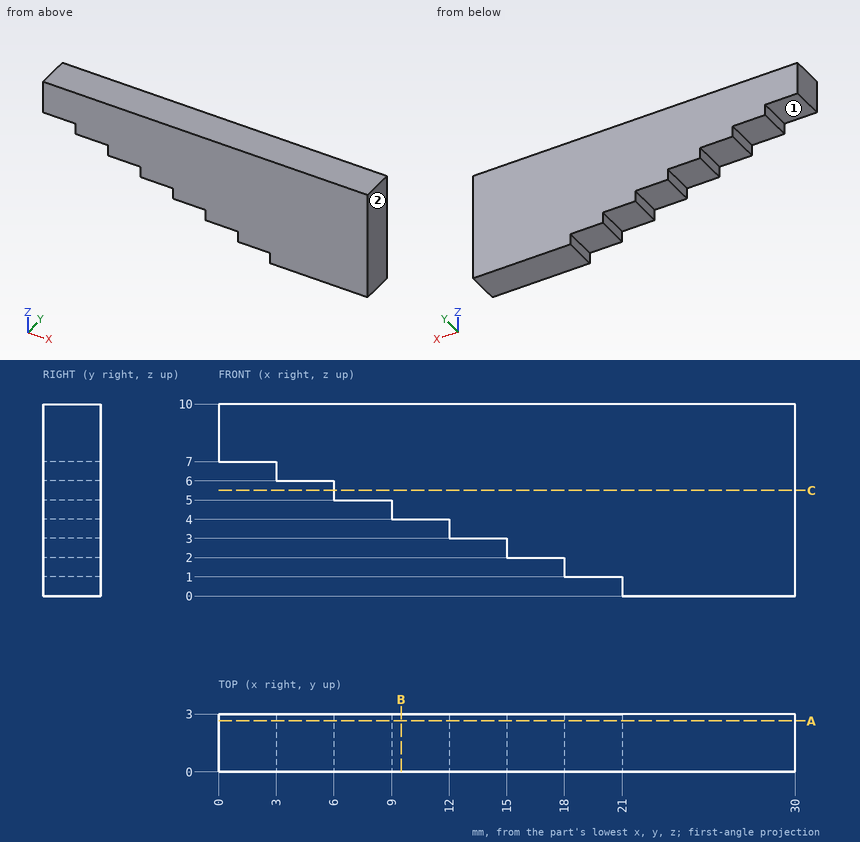
Verification items for this drawing (mm, ordinates from the low corner). A direction names the side the tool comes from. Round coordinates to 2 decimals unless told otherwise and drop trailing zeros. Loops run counter-clockwise (first coordinate to the right, second up) from the corner with the lowest first, then second, coordinate; pieces in that order, holes last. Notation, with made-up numbers: M 14,-20.75 L 47,-20.75 A12 cw 47,-11.75 Z; hole C 84,21 d4. An arc over 180 degrees is marked long. Answer as a JSON object with one key per item and string values.
1. Section check C-C (z = 5.5). Record the boundary of the cut face in (x, y), plus the area to 3 significant figures.
Reply:
{"outline": "M 6,0 L 30,0 L 30,3 L 6,3 Z", "area": "72.0 mm²"}
2. Scan lines: line 1 (X direction, y = 1.6, z = 3.5); line 2 (Z direction, x = 5.75, y = 2.05); line 3 (X direction, y = 1.5, z = 1.75). Record each from-to range of solid material in increasing order.
Reply:
{"line 1": "x = 12 to 30", "line 2": "z = 6 to 10", "line 3": "x = 18 to 30"}
3. Section check A-A (y = 2.65). Record the boundary of the cut face in (x, z), plus the area to 3 significant figures.
Reply:
{"outline": "M 0,7 L 3,7 L 3,6 L 6,6 L 6,5 L 9,5 L 9,4 L 12,4 L 12,3 L 15,3 L 15,2 L 18,2 L 18,1 L 21,1 L 21,0 L 30,0 L 30,10 L 0,10 Z", "area": "216 mm²"}
4. Gauge pin test, flat ends, axial feed: P1, Ø1.1, axis at y = 1, z = 5.5, coming from the -X side; P2, Ø1.1, axis at y = 1.5, z = 1.5, coming from the -X side; P3, Ø1.1, axis at y = 2, z = 3.5, coming from the -X side; P4, Ø3, axis at x = 24.5, z = 3, coming from the -Y side. Record the tip position at first contact, or that the pin passes through.
Reply:
{"P1": "stops at x = 3", "P2": "stops at x = 15", "P3": "stops at x = 9", "P4": "stops at y = 0"}
5. Access from +Z, -Z, +X, -X, +Y, -Y to the whole of each face (thin tool, end or side, straight path). Record for the marked faces 1 and 2.
Reply:
{"face 1": "-Z, -X, +Y, -Y", "face 2": "+Z, -Z, +X, +Y, -Y"}
6. Section check B-B (x = 9.5). Record the boundary of the cut face in (y, z).
Reply:
{"outline": "M 0,4 L 3,4 L 3,10 L 0,10 Z"}
